Build history of the part. All positions in model axes, mm. Round coordinates to 2 decimals unless told otherwise and drop trailing zeros. Loops run counter-clockwise (first coordinate to the right, second up) from the corner with the lowest first, then second, coordinate; pieces in that order, holes last. Notation, with made-up numbers: (57.25, 79) - (66.25, 79) arc R17 ccw to (66.25, 112) - close; hole circle Ø9 at (27.25, 88.25). An arc over 180 degrees is marked (long way). Answer as CSV lines item,"result". Start each with the question number.
Autodesk Inventor part; units mm, degrees
ref_plane "YZ Plane" through (0, 0, 0) normal (1, 0, 0) x (0, 1, 0)
ref_plane "XZ Plane" through (0, 0, 0) normal (0, 1, 0) x (-1, 0, 0)
ref_plane "XY Plane" through (0, 0, 0) normal (0, 0, 1) x (1, 0, 0)
sketch "Sketch1" plane through (0, 0, 0) normal (0, 1, 0) x (-1, 0, 0)
  arc A0 (-2.9651, 0.4562) -> (2.9651, 0.4562) centre (0, 0) ccw
  line L0 (0, 0) -> (0, 8)
  circle A1 centre (0, 8) radius 1.075
  line L1 (0, 8) -> (0, 13)
  circle A2 centre (0, 13) radius 1.075
  arc A3 (1.9942, 13.1525) -> (-1.9942, 13.1525) centre (0, 13) ccw
  line L2 (3, 0) -> (1.9942, 13.1525)
  line L3 (-3, 0) -> (-1.9942, 13.1525)
  circle A4 centre (0, 0) radius 2
  dimension "d0" = 6
  dimension "d1" = 8
  dimension "d2" = 2.15
  dimension "d3" = 5
  dimension "d4" = 2.15
  dimension "d5" = 4
  dimension "d6" = 4
extrude "Extrusion1" add sketch "Sketch1" against normal blind 1 contours L3 A3 L2 A0
properties part number "servoya giden parca"
Q1. Band-saw the part on D-D, the plane x = -1.6. List the corners of the cut face in (y, z), then the cut area to 3 significant figures.
Q2. Wall check: probe 1 along Z at (x, y) = (0, -0.55) (3 decimals); probe 2 along Z at (x, y) = (-0.55, -0.7); probe 3 along X at (y, z) = (-0.15, 0). Give the ranges that are in metal, low to high. Write a range as [from, to].
Q3. Band-saw the part on A-A, the plane z = 8. List the corners of the cut face in (x, y) (3 decimals).
Q4. Two-plate mould, pull along X, no slides. Class faces 1 (the cylindrical face through (0.23, -0.49, 11.95)), 2 (the flat face through (0, 0, 6)), 3 (the cylindrical face through (0, -0.5, 15)): released by +X, released by -X, zero draft, split by the parting line, or undercut.
Q5. Band-saw the part on C-C, the plane y = -0.7. Give the number of separate pieces and of enclosed holes in the cut face, then the cut area to 3 significant figures.
Q6. Band-saw the part on B-B, the plane x = 0. List the corners of the cut face in (y, z) (3 decimals).
Reported:
1,outline,"(-1, -2.54) - (0, -2.54) - (0, -1.2) - (-1, -1.2) - close; (-1, 1.2) - (0, 1.2) - (0, 14.2) - (-1, 14.2) - close"
1,area,"14.3 mm2"
2,probe 1,"z = [-3, -2], [2, 6.925], [9.075, 11.925], [14.075, 15]"
2,probe 2,"z = [-2.95, -1.92], [1.92, 7.08], [8.92, 12.08], [13.92, 14.92]"
2,probe 3,"x = [-3, -2], [2, 3]"
3,outline,"(-2.388, -1) - (-1.075, -1) - (-1.075, 0) - (-2.388, 0) - close; (1.075, -1) - (2.388, -1) - (2.388, 0) - (1.075, 0) - close"
4,face 1,"undercut"
4,face 2,"zero draft"
4,face 3,"split by the parting line"
5,separate pieces,"1"
5,enclosed holes,"3"
5,area,"65.7 mm2"
6,outline,"(-1, -3) - (0, -3) - (0, -2) - (-1, -2) - close; (-1, 2) - (0, 2) - (0, 6.925) - (-1, 6.925) - close; (-1, 9.075) - (0, 9.075) - (0, 11.925) - (-1, 11.925) - close; (-1, 14.075) - (0, 14.075) - (0, 15) - (-1, 15) - close"
